Print and shaded views of the part. All mm, measured from the part's lowest x, y and z. Round coordinates to 2 decimals unless told otherwise and drop trailing zeros. Order: outer loops, then holes, each group sorted by start corner. A loop starts at its lowest first (then second) coordinate and runs counter-clockwise, first axis right, second up.
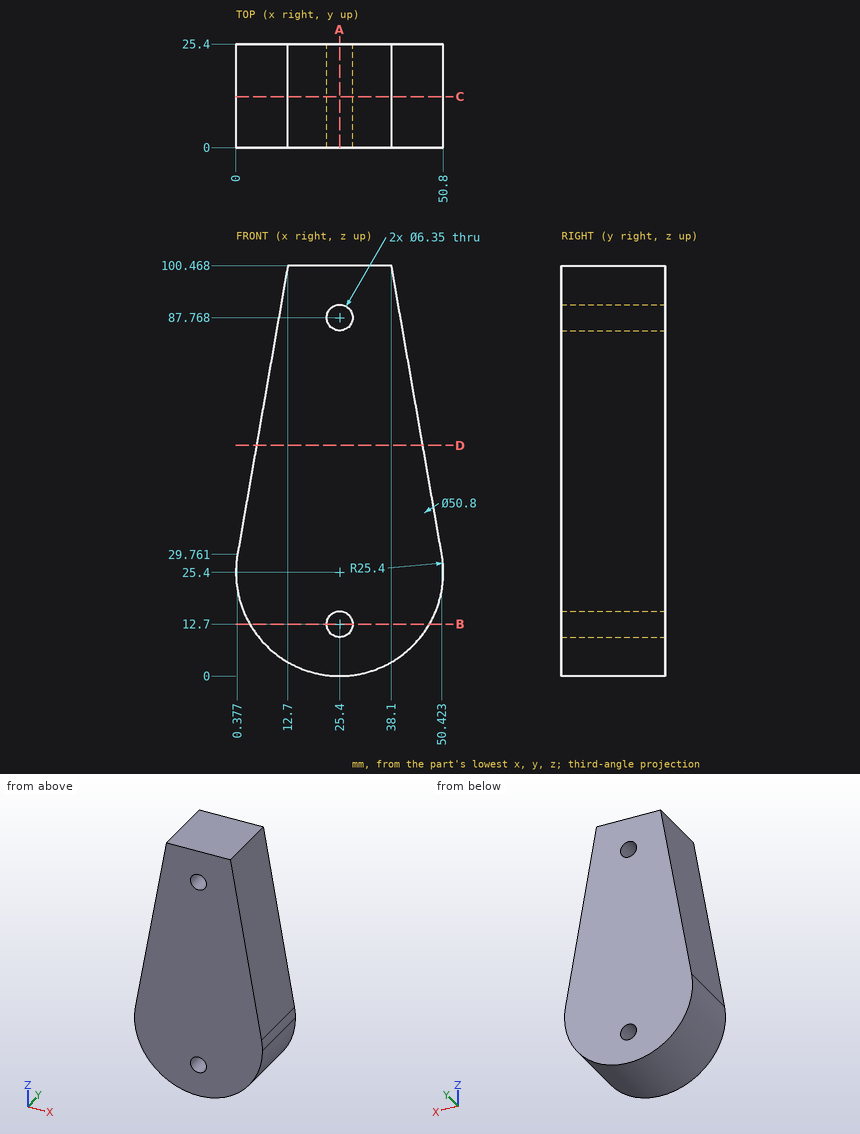
1. Pin check, flat tips, straight feed: P1, Ø3, axis at x = 29.5, y = 18, coming from the -Z side; P2, Ø5, axis at y = 16, z = 66, coming from the -X side; P3, Ø5, axis at y = 17, z = 62.5, coming from the -X side. Stop position of each tip, or through.
2. Cut at D-D, the plane z = 56.5. Write the cut outline in (x, y).
3. Cut at B-B, the plane z = 12.7. Write the cut outline in (x, y) (1 decimal).
4. Cut at A-A, the plane x = 25.4. Write the cut outline in (y, z) (1 decimal).
5. Cut at C-C, the plane y = 12.5. Give the number of separate pieces and of enclosed holes in the cut face, and give its area (3 significant figures).
6. Drill centre lines: line 1 (Z direction, x = 25.4, y = 7.25) (1 decimal); line 2 (X direction, y = 1.75, z = 32.5) (1 decimal); line 3 (Z direction, x = 36.5, y = 20.75) (1 decimal). Where is each one in solid material? Low to high.
Outcome:
1. P1: stops at z = 0.13
1. P2: stops at x = 6.26
1. P3: stops at x = 5.65
2. outline: (5.04, 0) - (45.76, 0) - (45.76, 25.4) - (5.04, 25.4) - close
3. outline: (3.4, 0) - (22.2, 0) - (22.2, 25.4) - (3.4, 25.4) - close; (28.6, 0) - (47.4, 0) - (47.4, 25.4) - (28.6, 25.4) - close
4. outline: (0, 0) - (25.4, 0) - (25.4, 9.5) - (0, 9.5) - close; (0, 15.9) - (25.4, 15.9) - (25.4, 84.6) - (0, 84.6) - close; (0, 90.9) - (25.4, 90.9) - (25.4, 100.5) - (0, 100.5) - close
5. separate pieces: 1
5. enclosed holes: 2
5. area: 3,840 mm2
6. line 1: z = 0 to 9.5, 15.9 to 84.6, 90.9 to 100.5
6. line 2: x = 0.9 to 49.9
6. line 3: z = 2.6 to 100.5
